Build history of the part. All positions in model axes, mm. Face numbers are marked on the shaded views. A direction names the side the tool comes from. Give positions to 0.01 mm unless a question says otherwise; leave off trailing zeros. Order: outer loops, then holes, each group sorted by start corner. A loop starts at its lowest first (then second) coordinate and runs counter-clockwise, first axis right, second up. Notation, with made-up numbers: (49, 34.5) - (58, 34.5) arc R25 cw to (58, 46.5) - close; hole circle Ø3 at (-37, 21). An arc over 180 degrees is marked (long way). Use a Markdown table: item, result. Add a question column.
(1) Slice it at D-D (y = 22). Write the cut outline in (x, z), then the cut area to 3 significant figures.
(2) Slice it at A-A (y = 1.5). Write the cut outline in (x, z), then the cut area to 3 significant figures.
(3) Flat gauge pins, fed straight in: pin 1 (12 mm diameter, centred on x = -7, z = 4.5, fed in from +Y); pin 2 (10 mm diameter, centred on x = 0.5, y = 7.5, fed in from +Z); pin 3 (1.3 mm diameter, centred on y = 8, z = 0, fed in from +X). Where does each tip first touch, or does it go through?
(4) Slice it at C-C (z = 5). Write the cut outline in (x, y), then the cut area to 3 significant figures.
(5) Wall check: line 1 (X direction, y = 20.5, z = -7.75); line 2 (X direction, y = -1.5, z = 5); line 3 (Z direction, x = -21.65, y = 15). Give the ranges that are in metal, low to high.
(6) Mould opens along X. For the marked faces 1, 2 and 3 say: +X half, -X half, draft (parallel to the pull), parting line (faces both ways), or undercut.
(7) Which spindle directions (+Z, -Z, +X, -X, +Y, -Y) get a long thin tool onto all of the face, cutting with end or side? Do the marked faces 4 and 5. Say none if no direction does.
(8) Slice it at B-B (x = 5). Write the cut outline in (y, z), then the cut area to 3 significant figures.
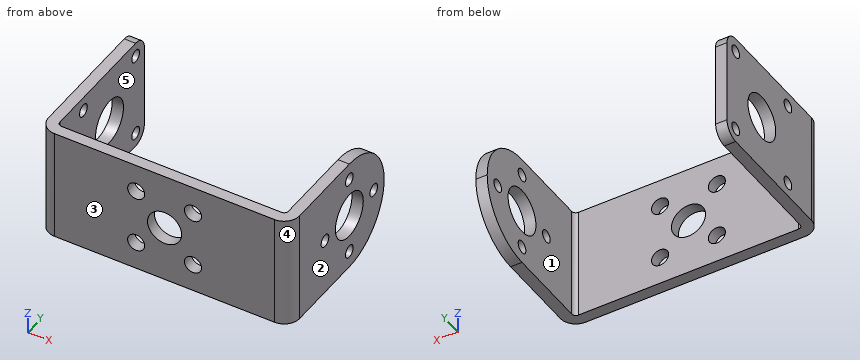
from build123d import *

# Parameters (mm, degrees)
SKETCH_1_W                         = 44.2
SKETCH_1_H                         = 20
SM_BASE_FLANGE_1_DEPTH             = 2
SM_EDGE_FLANGE_1_STRIP_W           = 9.4732
SM_EDGE_FLANGE_1_STRIP_H           = 2
SM_EDGE_FLANGE_1_STRIP_CUT_DEPTH   = 20
SM_EDGE_FLANGE_1_STRIP_2_W         = 9.4732
SM_EDGE_FLANGE_1_STRIP_2_H         = 2
SM_EDGE_FLANGE_1_STRIP_CUT_2_DEPTH = 20
SM_EDGE_FLANGE_1_DEPTH             = 20
SM_EDGE_FLANGE_1_BEND_DEPTH        = 20
CUT_EXTRUDE_1_REACH                = 53.756
SKETCH_14_R                        = 4
SKETCH_14_R_2                      = 1.1
CUT_EXTRUDE_2_REACH                = 53.756
SKETCH_15_R                        = 4
SKETCH_15_R_2                      = 1.1
FILLET_4_R                         = 2.5
FILLET_5_R                         = 2.5
CUT_EXTRUDE_3_REACH                = 38.296
SKETCH_16_R                        = 3
SKETCH_16_R_2                      = 1.5


# Sheet-metal steps are written as plain solids
with BuildPart() as part:
    # Sketch 1 → 基体-法兰1 (new body)
    with BuildSketch(Plane(origin=(0, 0, 0), x_dir=(1, 0, 0), z_dir=(0, 1, 0))):
        Rectangle(SKETCH_1_W, SKETCH_1_H)
    extrude(amount=-SM_BASE_FLANGE_1_DEPTH)

    # 边线-法兰1 strip (across the edge) → 边线-法兰1 strip cut (cut)
    with BuildSketch(Plane(origin=(-22.1, 0, -10), x_dir=(1, 0, 0), z_dir=(0, 0, 1))):
        with Locations((-2, -1)):
            Rectangle(SM_EDGE_FLANGE_1_STRIP_W, SM_EDGE_FLANGE_1_STRIP_H)
    extrude(amount=SM_EDGE_FLANGE_1_STRIP_CUT_DEPTH, mode=Mode.SUBTRACT)

    # 边线-法兰1 strip 2 (across the edge) → 边线-法兰1 strip cut 2 (cut)
    with BuildSketch(Plane(origin=(22.1, 0, 10), x_dir=(-1, 0, 0), z_dir=(0, 0, -1))):
        with Locations((-2, -1)):
            Rectangle(SM_EDGE_FLANGE_1_STRIP_2_W, SM_EDGE_FLANGE_1_STRIP_2_H)
    extrude(amount=SM_EDGE_FLANGE_1_STRIP_CUT_2_DEPTH, mode=Mode.SUBTRACT)

    # 边线-法兰1 section (across the edge) → 边线-法兰1 (add)
    with BuildSketch(Plane(origin=(-22.1, 0, -10), x_dir=(1, 0, 0), z_dir=(0, 0, 1))):
        with BuildLine():
            Line((0, 0.7366), (0, 25))
            Line((0, 25), (2, 25))
            Line((2, 25), (2, 0.7366))
            ThreePointArc((2, 0.7366), (2.215745145, 0.215745145), (2.7366, 0))
            Line((2.7366, 0), (2.7366, -2))
            ThreePointArc((2.7366, -2), (0.801531583, -1.198468417), (0, 0.7366))
        make_face()
    extrude(amount=SM_EDGE_FLANGE_1_DEPTH)

    # 边线-法兰1 section 2 (across the edge) → 边线-法兰1 bend (add)
    with BuildSketch(Plane(origin=(22.1, 0, 10), x_dir=(-1, 0, 0), z_dir=(0, 0, -1))):
        with BuildLine():
            Line((0, 0.7366), (0, 25))
            Line((0, 25), (2, 25))
            Line((2, 25), (2, 0.7366))
            ThreePointArc((2, 0.7366), (2.215745145, 0.215745145), (2.7366, 0))
            Line((2.7366, 0), (2.7366, -2))
            ThreePointArc((2.7366, -2), (0.801531583, -1.198468417), (0, 0.7366))
        make_face()
    extrude(amount=SM_EDGE_FLANGE_1_BEND_DEPTH)

    # 草图14 → 切除-拉伸1 (cut, up to next)
    with BuildSketch(Plane(origin=(22.1, 0, 0), x_dir=(0, 0, -1), z_dir=(1, 0, 0)), mode=Mode.PRIVATE) as cut_extrude_1_sk1:
        with BuildLine():
            ThreePointArc((-10, 15), (-7.071067812, 22.071067812), (0, 25))
            Line((0, 25), (-10, 25))
            Line((-10, 25), (-10, 15))
        make_face()
    cut_extrude_1_tool1 = extrude(cut_extrude_1_sk1.sketch, amount=-CUT_EXTRUDE_1_REACH, mode=Mode.PRIVATE) & part.part
    # 草图14 → 切除-拉伸1 (cut, up to next)
    with BuildSketch(Plane(origin=(22.1, 0, 0), x_dir=(0, 0, -1), z_dir=(1, 0, 0)), mode=Mode.PRIVATE) as cut_extrude_1_sk2:
        with BuildLine():
            ThreePointArc((0, 25), (7.071067812, 22.071067812), (10, 15))
            Line((10, 15), (10, 25))
            Line((10, 25), (0, 25))
        make_face()
    cut_extrude_1_tool2 = extrude(cut_extrude_1_sk2.sketch, amount=-CUT_EXTRUDE_1_REACH, mode=Mode.PRIVATE) & part.part
    # 草图14 → 切除-拉伸1 (cut, up to next)
    with BuildSketch(Plane(origin=(22.1, 0, 0), x_dir=(0, 0, -1), z_dir=(1, 0, 0)), mode=Mode.PRIVATE) as cut_extrude_1_sk3:
        with Locations(Location((0, 15, 0), (0, 0, 90))):
            Circle(SKETCH_14_R)
    cut_extrude_1_tool3 = extrude(cut_extrude_1_sk3.sketch, amount=-CUT_EXTRUDE_1_REACH, mode=Mode.PRIVATE) & part.part
    # 草图14 → 切除-拉伸1 (cut, up to next)
    with BuildSketch(Plane(origin=(22.1, 0, 0), x_dir=(0, 0, -1), z_dir=(1, 0, 0)), mode=Mode.PRIVATE) as cut_extrude_1_sk4:
        with Locations(Location((-7, 15, 0), (0, 0, 90))):
            Circle(SKETCH_14_R_2)
    cut_extrude_1_tool4 = extrude(cut_extrude_1_sk4.sketch, amount=-CUT_EXTRUDE_1_REACH, mode=Mode.PRIVATE) & part.part
    # 草图14 → 切除-拉伸1 (cut, up to next)
    with BuildSketch(Plane(origin=(22.1, 0, 0), x_dir=(0, 0, -1), z_dir=(1, 0, 0)), mode=Mode.PRIVATE) as cut_extrude_1_sk5:
        with Locations(Location((0, 22, 0), (0, 0, 90))):
            Circle(SKETCH_14_R_2)
    cut_extrude_1_tool5 = extrude(cut_extrude_1_sk5.sketch, amount=-CUT_EXTRUDE_1_REACH, mode=Mode.PRIVATE) & part.part
    # 草图14 → 切除-拉伸1 (cut, up to next)
    with BuildSketch(Plane(origin=(22.1, 0, 0), x_dir=(0, 0, -1), z_dir=(1, 0, 0)), mode=Mode.PRIVATE) as cut_extrude_1_sk6:
        with Locations(Location((7, 15, 0), (0, 0, 90))):
            Circle(SKETCH_14_R_2)
    cut_extrude_1_tool6 = extrude(cut_extrude_1_sk6.sketch, amount=-CUT_EXTRUDE_1_REACH, mode=Mode.PRIVATE) & part.part
    # 草图14 → 切除-拉伸1 (cut, up to next)
    with BuildSketch(Plane(origin=(22.1, 0, 0), x_dir=(0, 0, -1), z_dir=(1, 0, 0)), mode=Mode.PRIVATE) as cut_extrude_1_sk7:
        with Locations(Location((0, 8, 0), (0, 0, 90))):
            Circle(SKETCH_14_R_2)
    cut_extrude_1_tool7 = extrude(cut_extrude_1_sk7.sketch, amount=-CUT_EXTRUDE_1_REACH, mode=Mode.PRIVATE) & part.part
    add(cut_extrude_1_tool1.solids().sort_by_distance((22.1, 22.766321, 7.766321))[0], mode=Mode.SUBTRACT)
    add(cut_extrude_1_tool2.solids().sort_by_distance((22.1, 22.766321, -7.766321))[0], mode=Mode.SUBTRACT)
    add(cut_extrude_1_tool3.solids().sort_by_distance((22.1, 15, 0))[0], mode=Mode.SUBTRACT)
    add(cut_extrude_1_tool4.solids().sort_by_distance((22.1, 15, 7))[0], mode=Mode.SUBTRACT)
    add(cut_extrude_1_tool5.solids().sort_by_distance((22.1, 22, 0))[0], mode=Mode.SUBTRACT)
    add(cut_extrude_1_tool6.solids().sort_by_distance((22.1, 15, -7))[0], mode=Mode.SUBTRACT)
    add(cut_extrude_1_tool7.solids().sort_by_distance((22.1, 8, 0))[0], mode=Mode.SUBTRACT)

    # 草图15 → 切除-拉伸2 (cut, up to next)
    with BuildSketch(Plane.ZY.offset(22.1), mode=Mode.PRIVATE) as cut_extrude_2_sk1:
        with Locations(Location((0, 15, 0), (0, 0, 90))):
            Circle(SKETCH_15_R)
    cut_extrude_2_tool1 = extrude(cut_extrude_2_sk1.sketch, amount=-CUT_EXTRUDE_2_REACH, mode=Mode.PRIVATE) & part.part
    # 草图15 → 切除-拉伸2 (cut, up to next)
    with BuildSketch(Plane.ZY.offset(22.1), mode=Mode.PRIVATE) as cut_extrude_2_sk2:
        with Locations(Location((-7.5, 22.5, 0), (0, 0, 270))):
            Circle(SKETCH_15_R_2)
    cut_extrude_2_tool2 = extrude(cut_extrude_2_sk2.sketch, amount=-CUT_EXTRUDE_2_REACH, mode=Mode.PRIVATE) & part.part
    # 草图15 → 切除-拉伸2 (cut, up to next)
    with BuildSketch(Plane.ZY.offset(22.1), mode=Mode.PRIVATE) as cut_extrude_2_sk3:
        with Locations(Location((-7.5, 7.5, 0), (0, 0, 270))):
            Circle(SKETCH_15_R_2)
    cut_extrude_2_tool3 = extrude(cut_extrude_2_sk3.sketch, amount=-CUT_EXTRUDE_2_REACH, mode=Mode.PRIVATE) & part.part
    # 草图15 → 切除-拉伸2 (cut, up to next)
    with BuildSketch(Plane.ZY.offset(22.1), mode=Mode.PRIVATE) as cut_extrude_2_sk4:
        with Locations(Location((7.5, 7.5, 0), (0, 0, 270))):
            Circle(SKETCH_15_R_2)
    cut_extrude_2_tool4 = extrude(cut_extrude_2_sk4.sketch, amount=-CUT_EXTRUDE_2_REACH, mode=Mode.PRIVATE) & part.part
    # 草图15 → 切除-拉伸2 (cut, up to next)
    with BuildSketch(Plane.ZY.offset(22.1), mode=Mode.PRIVATE) as cut_extrude_2_sk5:
        with Locations(Location((7.5, 22.5, 0), (0, 0, 270))):
            Circle(SKETCH_15_R_2)
    cut_extrude_2_tool5 = extrude(cut_extrude_2_sk5.sketch, amount=-CUT_EXTRUDE_2_REACH, mode=Mode.PRIVATE) & part.part
    add(cut_extrude_2_tool1.solids().sort_by_distance((-22.1, 15, 0))[0], mode=Mode.SUBTRACT)
    add(cut_extrude_2_tool2.solids().sort_by_distance((-22.1, 22.5, -7.5))[0], mode=Mode.SUBTRACT)
    add(cut_extrude_2_tool3.solids().sort_by_distance((-22.1, 7.5, -7.5))[0], mode=Mode.SUBTRACT)
    add(cut_extrude_2_tool4.solids().sort_by_distance((-22.1, 7.5, 7.5))[0], mode=Mode.SUBTRACT)
    add(cut_extrude_2_tool5.solids().sort_by_distance((-22.1, 22.5, 7.5))[0], mode=Mode.SUBTRACT)

    # 圆角4
    fillet_4_edges = [part.edges().sort_by_distance(p)[0] for p in [
        (-21.1, 25, -10),
    ]]
    fillet(fillet_4_edges, radius=FILLET_4_R)

    # 圆角5
    fillet_5_edges = [part.edges().sort_by_distance(p)[0] for p in [
        (-21.1, 25, 10),
    ]]
    fillet(fillet_5_edges, radius=FILLET_5_R)

    # 草图16 → 切除-拉伸3 (cut, up to next)
    with BuildSketch(Plane.XZ.offset(2), mode=Mode.PRIVATE) as cut_extrude_3_sk1:
        with Locations(Location((0, 0, 0), (0, 0, 270))):
            Circle(SKETCH_16_R)
    cut_extrude_3_tool1 = extrude(cut_extrude_3_sk1.sketch, amount=-CUT_EXTRUDE_3_REACH, mode=Mode.PRIVATE) & part.part
    # 草图16 → 切除-拉伸3 (cut, up to next)
    with BuildSketch(Plane.XZ.offset(2), mode=Mode.PRIVATE) as cut_extrude_3_sk2:
        with Locations(Location((-5, 5, 0), (0, 0, 270))):
            Circle(SKETCH_16_R_2)
    cut_extrude_3_tool2 = extrude(cut_extrude_3_sk2.sketch, amount=-CUT_EXTRUDE_3_REACH, mode=Mode.PRIVATE) & part.part
    # 草图16 → 切除-拉伸3 (cut, up to next)
    with BuildSketch(Plane.XZ.offset(2), mode=Mode.PRIVATE) as cut_extrude_3_sk3:
        with Locations(Location((5, 5, 0), (0, 0, 270))):
            Circle(SKETCH_16_R_2)
    cut_extrude_3_tool3 = extrude(cut_extrude_3_sk3.sketch, amount=-CUT_EXTRUDE_3_REACH, mode=Mode.PRIVATE) & part.part
    # 草图16 → 切除-拉伸3 (cut, up to next)
    with BuildSketch(Plane.XZ.offset(2), mode=Mode.PRIVATE) as cut_extrude_3_sk4:
        with Locations(Location((5, -5, 0), (0, 0, 270))):
            Circle(SKETCH_16_R_2)
    cut_extrude_3_tool4 = extrude(cut_extrude_3_sk4.sketch, amount=-CUT_EXTRUDE_3_REACH, mode=Mode.PRIVATE) & part.part
    # 草图16 → 切除-拉伸3 (cut, up to next)
    with BuildSketch(Plane.XZ.offset(2), mode=Mode.PRIVATE) as cut_extrude_3_sk5:
        with Locations(Location((-5, -5, 0), (0, 0, 270))):
            Circle(SKETCH_16_R_2)
    cut_extrude_3_tool5 = extrude(cut_extrude_3_sk5.sketch, amount=-CUT_EXTRUDE_3_REACH, mode=Mode.PRIVATE) & part.part
    add(cut_extrude_3_tool1.solids().sort_by_distance((0, -2, 0))[0], mode=Mode.SUBTRACT)
    add(cut_extrude_3_tool2.solids().sort_by_distance((-5, -2, 5))[0], mode=Mode.SUBTRACT)
    add(cut_extrude_3_tool3.solids().sort_by_distance((5, -2, 5))[0], mode=Mode.SUBTRACT)
    add(cut_extrude_3_tool4.solids().sort_by_distance((5, -2, -5))[0], mode=Mode.SUBTRACT)
    add(cut_extrude_3_tool5.solids().sort_by_distance((-5, -2, -5))[0], mode=Mode.SUBTRACT)


solid = part.part
Solution:
| question | item | result |
|---|---|---|
| 1 | outline | (-22.1, -10) - (-20.1, -10) - (-20.1, -8.48) - (-22.1, -8.48) - close; (-22.1, -6.52) - (-20.1, -6.52) - (-20.1, 6.52) - (-22.1, 6.52) - close; (-22.1, 8.48) - (-20.1, 8.48) - (-20.1, 10) - (-22.1, 10) - close; (20.1, -7.14) - (22.1, -7.14) - (22.1, -1.1) - (20.1, -1.1) - close; (20.1, 1.1) - (22.1, 1.1) - (22.1, 7.14) - (20.1, 7.14) - close |
| 1 | area | 56.3 mm2 |
| 2 | outline | (-22.1, -10) - (-20.1, -10) - (-20.1, 10) - (-22.1, 10) - close; (20.1, -10) - (22.1, -10) - (22.1, 10) - (20.1, 10) - close |
| 2 | area | 80.0 mm2 |
| 3 | pin 1 | y = 0 |
| 3 | pin 2 | through |
| 3 | pin 3 | x = -20.1 |
| 4 | outline | (-22.1, 0.74) arc R2.74 ccw to (-19.36, -2) - (-6.5, -2) - (-6.5, 0) - (-19.36, 0) arc R0.74 cw to (-20.1, 0.74) - (-20.1, 25) - (-22.1, 25) - close; (-3.5, -2) - (3.5, -2) - (3.5, 0) - (-3.5, 0) - close; (6.5, -2) - (19.36, -2) arc R2.74 ccw to (22.1, 0.74) - (22.1, 23.66) - (20.1, 23.66) - (20.1, 0.74) arc R0.74 cw to (19.36, 0) - (6.5, 0) - close |
| 4 | area | 171 mm2 |
| 5 | line 1 | -22.1 to -20.1, 20.1 to 22.1 |
| 5 | line 2 | -20.94 to -6.5, -3.5 to 3.5, 6.5 to 20.94 |
| 5 | line 3 | -10 to -4, 4 to 10 |
| 6 | face 1 | undercut |
| 6 | face 2 | +X half |
| 6 | face 3 | draft |
| 7 | face 4 | +Z, -Z, +X, -Y |
| 7 | face 5 | +Z, -Z, +Y |
| 8 | outline | (-2, -10) - (0, -10) - (0, -6.5) - (-2, -6.5) - close; (-2, -3.5) - (0, -3.5) - (0, 3.5) - (-2, 3.5) - close; (-2, 6.5) - (0, 6.5) - (0, 10) - (-2, 10) - close |
| 8 | area | 28.0 mm2 |
